Study the drawing (mm; zero at the part's minimum x, y, z) and answer. Give positions to 0.01 mm unless a question says otherwise; leave off trailing zeros. Loops run counter-clockwise (first coordinate to the right, second up) from the corner with the lowest first, then second, coordinate; pieces in that order, holes last. Notation, with made-up numbers: M 22.5,77 L 37.5,77 A27 ccw 37.5,113 Z; hole C -27,-3.75 d1. An arc over 180 degrees is marked long. Return JSON: item names as keys, results as strings.
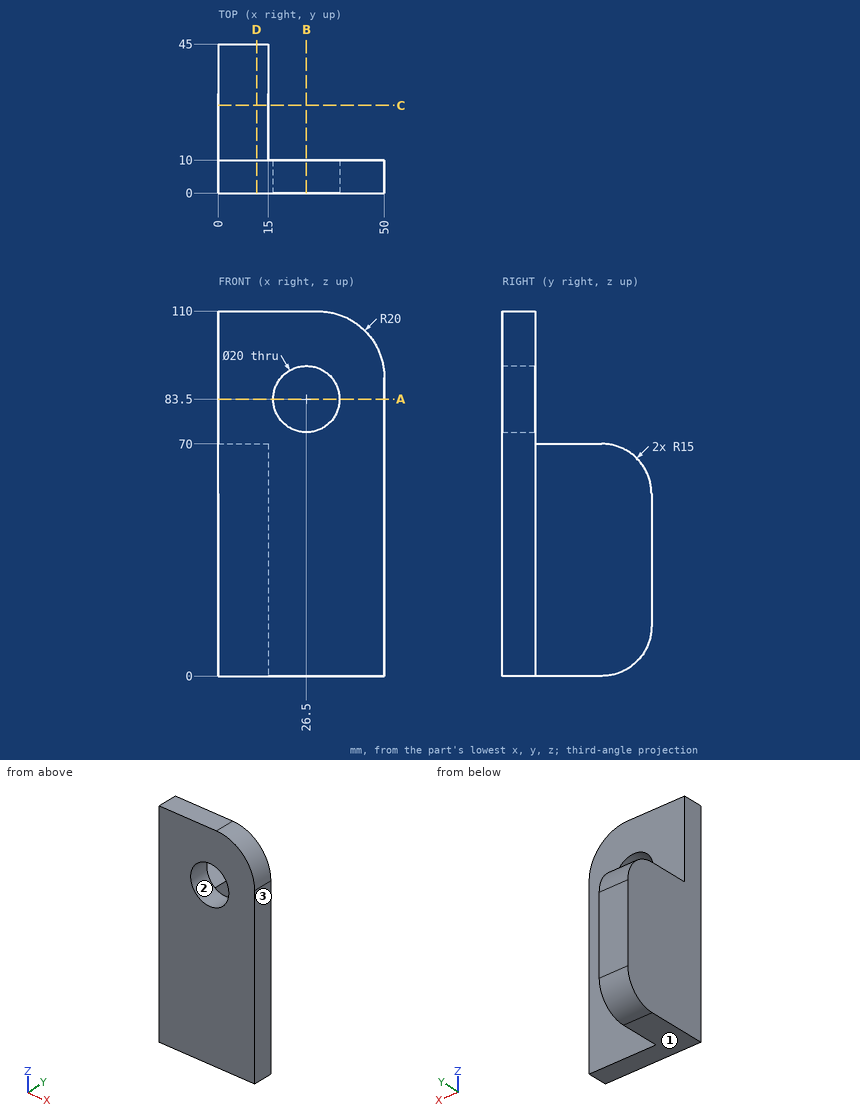
(1) The part is cut by section A-A (z = 83.5). Determine the outline of the cut face in (x, y), and give its area (3 significant figures).
Values follow:
{"outline": "M 0,0 L 16.5,0 L 16.5,10 L 0,10 Z; M 36.5,0 L 50,0 L 50,10 L 36.5,10 Z", "area": "300 mm²"}
(2) The part is cut by section B-B (x = 26.5). Determine the outline of the cut face in (y, z).
Values follow:
{"outline": "M 0,0 L 10,0 L 10,73.5 L 0,73.5 Z; M 0,93.5 L 10,93.5 L 10,110 L 0,110 Z"}
(3) Given pin 1 (16.5 mm diameter, centred on x = 11, y = 20, fed in from +Z); pin 2 (8 mm diameter, centred on x = 30, z = 18, fed in from +Y); pin 3 (12 mm diameter, centred on x = 26, y = 18, fed in from +Z), each flat-ended and moving along its own axis, determine where each tip first touches the part or whether it passes through.
Values follow:
{"pin 1": "z = 70", "pin 2": "y = 10", "pin 3": "through"}
(4) The part is cut by section C-C (y = 26.5). Determine the outline of the cut face in (x, z), and give its area (3 significant figures).
Values follow:
{"outline": "M 0,0 L 15,0 L 15,70 L 0,70 Z", "area": "1,050 mm²"}
(5) Straight lines are drawn through the part: line 1 along Z through (x, y) = (26.5, 4.5); line 2 along Y through (x, z) = (36, 49.5); line 3 along X through (y, z) = (24.5, 65). For each, find the intervals that lie inside material, in ascending order.
Values follow:
{"line 1": "0 to 73.5, 93.5 to 110", "line 2": "0 to 10", "line 3": "0 to 15"}
(6) Determine the mould class of the marked faces 1, 2 and 3 for opening direction X: released by +X, released by -X, zero draft, split by the parting line, or undercut.
Values follow:
{"face 1": "zero draft", "face 2": "undercut", "face 3": "released by +X"}
(7) The part is cut by section D-D (x = 11.5). Determine the outline of the cut face in (y, z).
Values follow:
{"outline": "M 0,0 L 30,0 A15 ccw 45,15 L 45,55 A15 ccw 30,70 L 10,70 L 10,110 L 0,110 Z"}
